Here's how the part is built. I have some questions about the finished solid (model axes, mm). Face numbers are marked on the shaded views. A direction names the side the tool comes from. Give positions to 0.01 mm unless a question says otherwise; leave off trailing zeros. Write each loop counter-clockwise with the first axis right and the second up, starting at its lowest first coordinate (ties: lowest second). Pieces come first, ordered by that corner, then holes. Notation, with made-up numbers: (75.5, -31.5) -> (131.5, -31.5) arc R23 ccw to (131.5, -11.5) -> close; hole circle Ø8 at (29, 72). An arc over 180 degrees is marked (long way). Return JSON: item names as keys, results as strings.
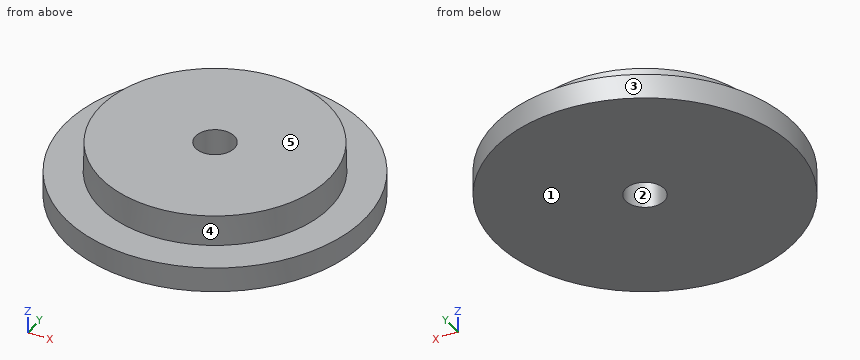
from build123d import *

# Parameters (mm, degrees)
F0_R     = 61.3
F1_DEPTH = 10.2
F2_R     = 47
F3_DEPTH = 12.5
F4_SIZE2 = 12.49999
F4_SIZE  = 0.27999
F5_R     = 7.9375
F6_DEPTH = 22.701


# Not quite as in the source:
# - a fillet or chamfer is up to 0.001 mm smaller than in the source, because OpenCascade refuses the exact size


with BuildPart() as f1:
    # F0 (on Top) → F1 (new body)
    with BuildSketch(Plane.XY):
        Circle(F0_R)
    extrude(amount=F1_DEPTH)

    # F2 (on face) → F3 (join)
    with BuildSketch(Plane.XY.offset(10.2)):
        Circle(F2_R)
    extrude(amount=F3_DEPTH)

    # F4 (size 0.28 and 12.5 in the source; OpenCascade refuses exactly that, so slightly less here)
    f4_edges = [f1.edges().sort_by_distance(p)[0] for p in [
        (-47, 0, 22.7),
    ]]
    f4_side = f1.faces().sort_by_distance((0, 0, 22.7))[0]
    chamfer(f4_edges, length=F4_SIZE, length2=F4_SIZE2, reference=f4_side)

    # F5 (on face) → F6 (cut, through all)
    with BuildSketch(Plane.XY.offset(22.7)):
        Circle(F5_R)
    extrude(amount=-F6_DEPTH, mode=Mode.SUBTRACT)


solid = f1.part
1. Suppose I cut it at C-C, the plane z = 1.75. List the corners of the cut face in (x, y) for me (1 decimal), and give its area (3 significant figures).
Taken from the geometry:
{"outline": "circle Ø122.6 at (0, 0); hole circle Ø15.9 at (0, 0)", "area": "11,600 mm²"}
2. Suppose I cut it at D-D, the plane z = 19.25. List the corners of the cut face in (x, y) for me (1 decimal), and give its area (3 significant figures).
Taken from the geometry:
{"outline": "circle Ø93.6 at (0, 0); hole circle Ø15.9 at (0, 0)", "area": "6,680 mm²"}
3. For pin 1 Ø2 at (y, z) = (-22.5, 8) entering from +X; pin 2 Ø5 at (x, y) = (-2, 23.5) entering from -Z; pin 3 Ø10 at (x, z) = (-28.5, 5) entering from +Y; pin 4 Ø6 at (x, z) = (18, 4.5) entering from -Y, each with a flat end and sliding along its axis, tell me the tip position at first contact or that it passes through.
Taken from the geometry:
{"pin 1": "stops at x = 57.41", "pin 2": "stops at z = 0", "pin 3": "stops at y = 56.62", "pin 4": "stops at y = -59.44"}
4. Which directions (+Z, -Z, +X, -X, +Y, -Y) give clear straight access to the entire face, cutting with the end or side of a thin tool? Please do the marked faces 4 and 5.
Taken from the geometry:
{"face 4": "+Z", "face 5": "+Z, +X, -X, +Y, -Y"}
5. If we mould it in two halves opening along Y, with no side actions, what happens to the marked faces 1, 2 and 3? For each: released by +Y, released by -Y, zero draft, split by the parting line, or undercut.
Taken from the geometry:
{"face 1": "zero draft", "face 2": "undercut", "face 3": "split by the parting line"}
6. If I drill on line 1 (Y direction, x = 0, z = 8); line 2 (X direction, y = 0.5, z = 21.75); line 3 (Z direction, x = 27.5, y = -51.5), over which ranges is the centre line in solid material (lowest first)? Write a range as [from, to].
Taken from the geometry:
{"line 1": "y = [-61.3, -7.94], [7.94, 61.3]", "line 2": "x = [-46.74, -7.92], [7.92, 46.74]", "line 3": "z = [0, 10.2]"}
